Check sheet for the modelled part. Datum: model origin and axes. Units: mm. Give positions to 0.01 mm unless a question says otherwise; leave off trailing zeros. Loops run counter-clockwise (first coordinate to the right, second up) from the corner with the lowest first, then second, coordinate; pieces in that order, holes last. Notation, with made-up numbers: (78.25, -37.5) -> (125.25, -37.5) arc R19 cw to (125.25, -24.5) -> close; hole circle Ø2 at (67.25, -20.5). An arc over 180 degrees is marked (long way). Write each question's results on one line, items separated by ' | '. Start each with the question number.
1. Cross-section at B-B on z = 2.8. Count the separate pieces of the cut face and the enclosed holes in it, and give its area (3 significant figures).
2. Cross-section at D-D on x = 100.5. Record the boundary of the cut face in (y, z), and give its area (3 significant figures).
3. Gauge pin test, flat ends, axial feed: pin 1 Ø1.5 at (x, z) = (-114.5, 2.5) entering from +Y; pin 2 Ø3 at (x, z) = (-75.5, 3) entering from -Y; pin 3 Ø2.5 at (x, z) = (-10, 1.5) entering from -Y. Record the tip position at first contact, or that the pin passes through.
4. Material ranges on L1, parallel to X at y = 25.5, z = 4.5; L2, parallel to Y at x = 3.5, z = 3.65; L3, parallel to X at y = -87, z = 3.4, recorded low to high. Write a range as from..to.
5. Cross-section at A-A on y = 7.5. Record the boundary of the cut face in (x, z).
6. Cross-section at C-C on x = 22.5. Record the boundary of the cut face in (y, z), and give its area (3 significant figures).
from build123d import *

# Parameters (mm, degrees)
SKETCH1_W           = 26.358753283
SKETCH1_H           = 29.759882739
BOSS_EXTRUDE1_DEPTH = 5


with BuildPart() as part:
    # Sketch1 → Boss-Extrude1 (new body)
    with BuildSketch(Plane.XY):
        with BuildLine():
            Line((-133.705700246, -95.388044307), (-107.275003874, -95.388044307))
            ThreePointArc((-107.275003874, -95.388044307), (-103.044823488, -97.722416069), (-98.814643102, -95.388044307))
            Line((-98.814643102, -95.388044307), (-77.510422411, -95.388044307))
            Line((-77.510422411, -95.388044307), (-60.765070658, -66.384244279))
            ThreePointArc((-60.765070658, -66.384244279), (-58.284996417, -64.588629688), (-57.969985686, -61.543015096))
            Line((-57.969985686, -61.543015096), (-42.86940626, -35.388044307))
            Line((-42.86940626, -35.388044307), (31.031428196, -35.388044307))
            Line((31.031428196, -35.388044307), (46.120827825, -61.523651119))
            ThreePointArc((46.120827825, -61.523651119), (46.354900962, -64.791664092), (49.068046647, -66.628383861))
            Line((49.068046647, -66.628383861), (65.672444348, -95.388044307))
            Line((65.672444348, -95.388044307), (86.685893367, -95.388044307))
            ThreePointArc((86.685893367, -95.388044307), (91.206010968, -98.250630713), (95.726128569, -95.388044307))
            Line((95.726128569, -95.388044307), (121.578619423, -95.388044307))
            ThreePointArc((121.578619423, -95.388044307), (126.098737025, -98.250630713), (130.618854626, -95.388044307))
            Line((130.618854626, -95.388044307), (151.632303645, -95.388044307))
            Line((151.632303645, -95.388044307), (151.632303645, 95.46540018))
            Line((151.632303645, 95.46540018), (75.512150198, 95.46540018))
            ThreePointArc((75.512150198, 95.46540018), (71.182023179, 97.96540018), (66.85189616, 95.46540018))
            Line((66.85189616, 95.46540018), (-78.689780736, 95.46540018))
            ThreePointArc((-78.689780736, 95.46540018), (-83.019907754, 97.96540018), (-87.350034773, 95.46540018))
            Line((-87.350034773, 95.46540018), (-163.470281709, 95.46540018))
            Line((-163.470281709, 95.46540018), (-163.470281709, -95.388044307))
            Line((-163.470281709, -95.388044307), (-142.166061018, -95.388044307))
            ThreePointArc((-142.166061018, -95.388044307), (-137.935880632, -97.722416069), (-133.705700246, -95.388044307))
        make_face()
        with Locations((-26.546016438, 12.255373732)):
            Rectangle(SKETCH1_W, SKETCH1_H, mode=Mode.SUBTRACT)
        with Locations((14.708131863, 12.255373732)):
            Rectangle(SKETCH1_W, SKETCH1_H, mode=Mode.SUBTRACT)
    extrude(amount=BOSS_EXTRUDE1_DEPTH)


solid = part.part
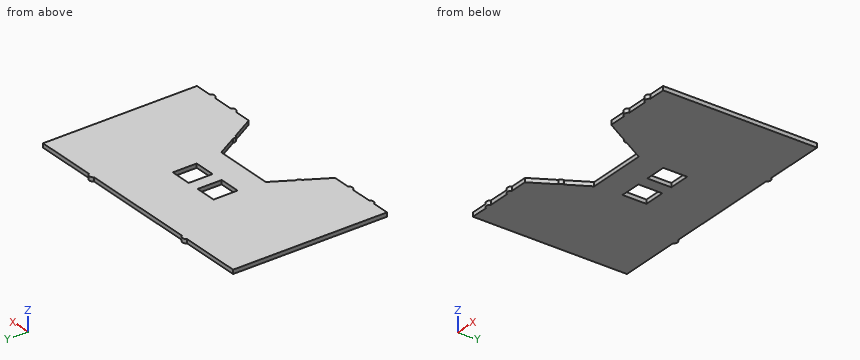
Geometry says:
1) separate pieces: 1 | enclosed holes: 2 | area: 52,200 mm^2
2) outline: (-95.39, 0) -> (95.47, 0) -> (95.47, 5) -> (-95.39, 5) -> close | area: 954 mm^2
3) pin 1: y = 95.47 | pin 2: y = -94.5 | pin 3: y = -35.39
4) L1: -163.47..-39.73, -13.37..1.53, 27.89..151.63 | L2: -35.39..-2.62, 27.14..95.47 | L3: -163.47..-72.67, 60.83..151.63
5) outline: (-163.47, 0) -> (-39.73, 0) -> (-39.73, 5) -> (-163.47, 5) -> close; (-13.37, 0) -> (1.53, 0) -> (1.53, 5) -> (-13.37, 5) -> close; (27.89, 0) -> (151.63, 0) -> (151.63, 5) -> (27.89, 5) -> close
6) outline: (-35.39, 0) -> (-2.62, 0) -> (-2.62, 5) -> (-35.39, 5) -> close; (27.14, 0) -> (95.47, 0) -> (95.47, 5) -> (27.14, 5) -> close | area: 505 mm^2
